```python
from build123d import *

# Parameters (mm, degrees)
SKETCH1_R           = 1.35
BOSS_EXTRUDE1_DEPTH = 1.6
SKETCH2_W           = 7.53328877
SKETCH2_H           = 5.48663035
BOSS_EXTRUDE2_DEPTH = 3.2
SKETCH3_W           = 8.985946342
SKETCH3_H           = 6.956967826
BOSS_EXTRUDE3_DEPTH = 3
SKETCH4_W           = 8.28060663
SKETCH4_H           = 15.055648418
BOSS_EXTRUDE4_DEPTH = 6
SKETCH5_W           = 16.070010529
SKETCH5_H           = 11.93886501
BOSS_EXTRUDE5_DEPTH = 16
SKETCH6_W           = 19.440745211
SKETCH6_H           = 12.150465756
BOSS_EXTRUDE6_DEPTH = 13.5
SKETCH7_W           = 18.225698636
SKETCH7_H           = 15.309586854
BOSS_EXTRUDE7_DEPTH = 2.4
SKETCH8_W           = 50.998692198
SKETCH8_H           = 4.375780892
BOSS_EXTRUDE8_DEPTH = 8.5
SKETCH9_W           = 1.831399212
SKETCH9_H           = 15.719207136
BOSS_EXTRUDE9_DEPTH = 5.5


with BuildPart() as part:
    # Sketch1 → Boss-Extrude1 (new body)
    with BuildSketch(Plane(origin=(0, 0, 0), x_dir=(1, 0, 0), z_dir=(0, 1, 0))):
        with BuildLine():
            Line((-39.5, -28), (39.5, -28))
            ThreePointArc((39.5, -28), (41.621320344, -27.121320344), (42.5, -25))
            Line((42.5, -25), (42.5, 25))
            ThreePointArc((42.5, 25), (41.621320344, 27.121320344), (39.5, 28))
            Line((39.5, 28), (-39.5, 28))
            ThreePointArc((-39.5, 28), (-41.621320344, 27.121320344), (-42.5, 25))
            Line((-42.5, 25), (-42.5, -25))
            ThreePointArc((-42.5, -25), (-41.621320344, -27.121320344), (-39.5, -28))
        make_face()
        with Locations((-39, 24.5)):
            Circle(SKETCH1_R, mode=Mode.SUBTRACT)
        with Locations((19, 24.5)):
            Circle(SKETCH1_R, mode=Mode.SUBTRACT)
        with Locations((19, -24.5)):
            Circle(SKETCH1_R, mode=Mode.SUBTRACT)
        with Locations((-39, -24.5)):
            Circle(SKETCH1_R, mode=Mode.SUBTRACT)
    extrude(amount=BOSS_EXTRUDE1_DEPTH)

    # Sketch2 → Boss-Extrude2 (add)
    with BuildSketch(Plane(origin=(0, 1.6, 0), x_dir=(1, 0, 0), z_dir=(0, 1, 0))):
        with Locations((-31.3, -26.343842904)):
            Rectangle(SKETCH2_W, SKETCH2_H)
    extrude(amount=BOSS_EXTRUDE2_DEPTH)

    # Sketch3 → Boss-Extrude3 (add)
    with BuildSketch(Plane(origin=(0, 1.6, 0), x_dir=(1, 0, 0), z_dir=(0, 1, 0))):
        with Locations((-16.5, -25.555818694)):
            Rectangle(SKETCH3_W, SKETCH3_H)
        with Locations((-3, -25.555818694)):
            Rectangle(SKETCH3_W, SKETCH3_H)
    extrude(amount=BOSS_EXTRUDE3_DEPTH)

    # Sketch4 → Boss-Extrude4 (add)
    with BuildSketch(Plane(origin=(0, 1.6, 0), x_dir=(1, 0, 0), z_dir=(0, 1, 0))):
        with Locations((11.5, -22.720760552)):
            Rectangle(SKETCH4_W, SKETCH4_H)
    extrude(amount=BOSS_EXTRUDE4_DEPTH)

    # Sketch5 → Boss-Extrude5 (add)
    with BuildSketch(Plane(origin=(0, 1.6, 0), x_dir=(1, 0, 0), z_dir=(0, 1, 0))):
        with Locations((37.060775688, -19)):
            Rectangle(SKETCH5_W, SKETCH5_H)
        with Locations((37.060775688, -1)):
            Rectangle(SKETCH5_W, SKETCH5_H)
    extrude(amount=BOSS_EXTRUDE5_DEPTH)

    # Sketch6 → Boss-Extrude6 (add)
    with BuildSketch(Plane(origin=(0, 1.6, 0), x_dir=(1, 0, 0), z_dir=(0, 1, 0))):
        with Locations((36.574757039, 17.75)):
            Rectangle(SKETCH6_W, SKETCH6_H)
    extrude(amount=BOSS_EXTRUDE6_DEPTH)

    # Sketch7 → Boss-Extrude7 (add)
    with BuildSketch(Plane(origin=(0, 1.6, 0), x_dir=(1, 0, 0), z_dir=(0, 1, 0))):
        with Locations((-13.25, 4.5)):
            Rectangle(SKETCH7_W, SKETCH7_H)
    extrude(amount=BOSS_EXTRUDE7_DEPTH)

    # Sketch8 → Boss-Extrude8 (add)
    with BuildSketch(Plane(origin=(0, 1.6, 0), x_dir=(1, 0, 0), z_dir=(0, 1, 0))):
        with Locations((-10, 24.024952291)):
            Rectangle(SKETCH8_W, SKETCH8_H)
    extrude(amount=BOSS_EXTRUDE8_DEPTH)

    # Sketch9 → Boss-Extrude9 (add)
    with BuildSketch(Plane(origin=(0, 1.6, 0), x_dir=(1, 0, 0), z_dir=(0, 1, 0))):
        with Locations((-38.332266869, 0)):
            Rectangle(SKETCH9_W, SKETCH9_H)
    extrude(amount=BOSS_EXTRUDE9_DEPTH)


solid = part.part
```
Verification items for the finished model (mm, model axes). A direction names the side the tool comes from. Give positions to 0.01 mm unless a question says otherwise; leave off trailing zeros. Order: outer loops, then holes, each group sorted by start corner. A loop starts at its lowest first (then second) coordinate and runs counter-clockwise, first axis right, second up. Notation, with made-up numbers: (74, 20.25) - (83, 20.25) arc R25 ccw to (83, 44.25) - close; hole circle Ø2 at (-2.5, 70.5). An arc over 180 degrees is marked (long way). Answer as CSV lines item,"result". Start each with the question number.
Item 1: Mould release check, pull along X, two halves, no side actions. Record for faces 1 (the face through (44, 1.6, 1)), 2 (the face through (15.499, 6, -24)), 3 (the face through (-35.499, 6, -24)), 4 (the face through (45.096, 9, 1)): released by +X, released by -X, zero draft, split by the parting line, or undercut.
Item 2: Access from +Z, -Z, +X, -X, +Y, -Y to the whole of each face (thin tool, end or side, straight path). Record for faces 5 (the face through (11, 7.6, 23)), 6 (the face through (37, 9, 24.969)), 7 (the face through (37, 9, 6.969)), 8 (the face through (44, 1.6, -18)).
Item 3: Section check C-C, the plane z = -20. Record the boundary of the cut face in (x, y).
Item 4: Section check A-A, the plane y = 13.5. Record the boundary of the cut face in (x, z), plus the area to 3 significant figures.
Item 5: Section check B-B, the plane x = 19. Record the boundary of the cut face in (y, z), plus the area to 3 significant figures.
Item 6: Gauge pin test, flat ends, axial feed: pin 1 (5.5 mm diameter, centred on x = -15.5, z = 24.5, fed in from +Y); pin 2 (8 mm diameter, centred on x = 36.5, y = 2, fed in from +Z); pin 3 (3.5 mm diameter, centred on y = 9.5, z = 16.5, fed in from -X). Record the tip position at first contact, or that the pin passes through.
Item 7: Section check D-D, the plane x = -30. Record the boundary of the cut face in (y, z), plus the area to 3 significant figures.
Item 8: Material ranges on L1, parallel to Z at x = 19, y = 1; L2, parallel to X at y = 0.8, z = -24.5; L3, parallel to Z at x = -12.5, y = 2, recorded low to high.
Filled in:
1,face 1,"zero draft"
1,face 2,"undercut"
1,face 3,"released by -X"
1,face 4,"released by +X"
2,face 5,"+Z, -X, +Y"
2,face 6,"+Z, +X, +Y"
2,face 7,"+X, +Y"
2,face 8,"+Z, -Z, +X, -Y"
3,outline,"(-42.5, 0) - (42.5, 0) - (42.5, 1.6) - (46.3, 1.6) - (46.3, 15.1) - (26.85, 15.1) - (26.85, 1.6) - (-42.5, 1.6) - close"
4,outline,"(26.85, -23.83) - (46.3, -23.83) - (46.3, -11.67) - (26.85, -11.67) - close; (29.03, -4.97) - (45.1, -4.97) - (45.1, 6.97) - (29.03, 6.97) - close; (29.03, 13.03) - (45.1, 13.03) - (45.1, 24.97) - (29.03, 24.97) - close"
4,area,"620 mm^2"
5,outline,"(0, -28) - (1.6, -28) - (1.6, -25.85) - (0, -25.85) - close; (0, -23.15) - (1.6, -23.15) - (1.6, 23.15) - (0, 23.15) - close; (0, 25.85) - (1.6, 25.85) - (1.6, 28) - (0, 28) - close"
5,area,"81.0 mm^2"
6,pin 1,"y = 4.6"
6,pin 2,"z = 28"
6,pin 3,"x = 29.03"
7,outline,"(0, -28) - (1.6, -28) - (1.6, -26.21) - (10.1, -26.21) - (10.1, -21.84) - (1.6, -21.84) - (1.6, 23.6) - (4.8, 23.6) - (4.8, 29.09) - (1.6, 29.09) - (1.6, 28) - (0, 28) - close"
7,area,"144 mm^2"
8,L1,"-28 to -25.85, -23.15 to 23.15, 25.85 to 28"
8,L2,"-42.5 to -40.35, -37.65 to 17.65, 20.35 to 42.5"
8,L3,"-26.21 to -21.84, -12.15 to 3.15, 22.08 to 29.03"
